```python
from build123d import *
from build123d.topology import SkipClean

# Parameters (mm, degrees)
SKETCH2_R           = 13.49375
EXTRUDE1_DEPTH      = 23.495
SKETCH15_R          = 13.4874
BOSS_EXTRUDE1_DEPTH = 17.78
SKETCH16_R          = 7.7343
CUT_EXTRUDE1_DEPTH  = 46.47293924
SKETCH20_R          = 13.4874
BOSS_EXTRUDE2_DEPTH = 17.78
SKETCH22_R          = 13.335
BOSS_EXTRUDE3_DEPTH = 21.9075
BOSS_EXTRUDE3_TAPER = 1.75
CHAMFER1_SIZE       = 1.360714286
CHAMFER1_SIZE_2     = 1.404253042
SKETCH25_R          = 13.335
BOSS_EXTRUDE4_DEPTH = 21.9075
BOSS_EXTRUDE4_DRAFT = -15
SKETCH28_R          = 10.499412296
CUT_EXTRUDE6_DEPTH  = 21.9075
FILLET1_R           = 0.762
CIRPATTERN1_COUNT   = 2
CIRPATTERN1_ANGLE   = 180
SKETCH26_R          = 7.7343
CUT_EXTRUDE4_DEPTH  = 93.597306097
SKETCH29_R          = 7.7343
CUT_EXTRUDE7_DEPTH  = 59.850524324


with BuildPart() as part:
    # Sketch2 → Extrude1 (new body)
    with BuildSketch(Plane(origin=(-41.275, 0, 0), x_dir=(0, 0, -1), z_dir=(1, 0, 0))):
        with Locations(Location((0, 0, 0), (0, 0, 180))):
            Circle(SKETCH2_R)
    extrude(amount=EXTRUDE1_DEPTH)

    # Sketch5 → Cut-Revolve1 (revolve, cut)
    with BuildSketch(Plane.XY):
        Polygon((-36.995957679, 12.118934671), (-32.762624346, 12.118934671), (-31.387809017, 13.49375), (-41.275, 13.49375), (-41.275, 8.894445), align=None)
        Polygon((-17.78, 12.118934671), (-19.896666667, 12.118934671), (-21.271481995, 13.49375), (-17.78, 13.49375), align=None)
    revolve(axis=Axis((0, 0, 0), (-1, 0, 0)), mode=Mode.SUBTRACT)

    # Sketch15 → Boss-Extrude1 (add)
    with BuildSketch(Plane(origin=(-17.78, 0, 0), x_dir=(0, 0, -1), z_dir=(1, 0, 0))):
        Circle(SKETCH15_R)
    extrude(amount=BOSS_EXTRUDE1_DEPTH)

    # Sketch16 → Cut-Extrude1 (cut, through all)
    with BuildSketch(Plane(origin=(0, 0, 0), x_dir=(0, 0, -1), z_dir=(1, 0, 0))):
        Circle(SKETCH16_R)
    extrude(amount=-CUT_EXTRUDE1_DEPTH, mode=Mode.SUBTRACT)

    # Fillet1
    fillet1_edges = [part.edges().sort_by_distance(p)[0] for p in [
        (-17.78, 0, 13.4874),
    ]]
    fillet(fillet1_edges, radius=FILLET1_R)


with BuildPart() as body_2:
    # Sketch20 → Boss-Extrude2 (new body)
    with BuildSketch(Plane(origin=(0, 17.78, 0), x_dir=(-1, 0, 0), z_dir=(0, 1, 0))):
        with Locations(Location((0, 0, 0), (0, 0, 90))):
            Circle(SKETCH20_R)
    extrude(amount=-BOSS_EXTRUDE2_DEPTH)


with BuildPart() as body_3:
    # Sketch22 → Boss-Extrude3 (new body)
    with BuildSketch(Plane(origin=(0, 17.78, 0), x_dir=(-1, 0, 0), z_dir=(0, 1, 0))):
        Circle(SKETCH22_R)
    extrude(amount=BOSS_EXTRUDE3_DEPTH, taper=BOSS_EXTRUDE3_TAPER)

    # Chamfer1
    # the kernel refuses this chamfer: 1.404253042, 1.360714286 mm, written as the material it takes off along each edge
    with BuildSketch(Plane(origin=(0, 39.6875, 0), x_dir=(-1, 0, 0), z_dir=(0, 0, 1))) as chamfer1_piece_1:
        Polygon((12.665665338 + CHAMFER1_SIZE * 0.0305385132034, CHAMFER1_SIZE * 0.999533590627), (12.665665338 - CHAMFER1_SIZE_2, 0), (12.665665338, 0), align=None)
    revolve(axis=Axis((0, 39.6875, 0), (0, -1, 0)), mode=Mode.SUBTRACT)


with BuildPart() as boss_extrude4_tool:
    # Sketch25 → Boss-Extrude4 (with draft: the straight prism first)
    with BuildSketch(Plane.XZ.offset(-17.78)):
        Circle(SKETCH25_R)
    extrude(amount=-BOSS_EXTRUDE4_DEPTH)
    # Boss-Extrude4: the draft: its side faces are tilted about the plane it starts from
    boss_extrude4_sides = [boss_extrude4_tool.faces().sort_by_distance(p)[0] for p in [
        (-13.335, 28.73375, 0),
    ]]
    draft(boss_extrude4_sides, Plane.XZ.offset(-17.78), BOSS_EXTRUDE4_DRAFT)


with BuildPart() as body_3_1:
    add(body_3.part)

    # Boss-Extrude4: add boss_extrude4_tool
    add(boss_extrude4_tool.part)

    # Sketch28 → Cut-Extrude6 (cut)
    with BuildSketch(Plane(origin=(0, 39.6875, 0), x_dir=(1, 0, 0), z_dir=(0, 1, 0))):
        with Locations(Location((0, 0, 0), (0, 0, 270))):
            Circle(SKETCH28_R)
    extrude(amount=-CUT_EXTRUDE6_DEPTH, mode=Mode.SUBTRACT)


with BuildPart() as cirpattern1_1:
    # CirPattern1: pattern copy
    add(part.part.rotate(Axis((0, 0, 12.651043997), (0, 0, -1)), 1 * CIRPATTERN1_ANGLE / (CIRPATTERN1_COUNT - 1)))


with BuildPart() as part_1:
    add(part.part)

    # Combine2: union body 3, body 2, CirPattern1_1
    add(body_3_1.part)
    add(body_2.part)
    add(cirpattern1_1.part)

    # Sketch30 → Revolve1 (revolve)
    with SkipClean():  # the faces are left unmerged after this step: merging them gives an invalid solid
        with BuildSketch(Plane.XY, mode=Mode.PRIVATE) as revolve1_sk:
            with BuildLine():
                Line((0, 17.78), (0, 8.89))
                ThreePointArc((0, 8.89), (-7.214370781, 12.4003004), (-13.589, 17.272))
                Line((-13.589, 17.272), (-13.589, 17.78))
                Line((-13.589, 17.78), (0, 17.78))
            make_face()
        revolve(revolve1_sk.sketch.rotate(Axis((0, 17.78, 0), (0, -1, 0)), 270), axis=Axis((0, 17.78, 0), (0, -1, 0)))

    # Sketch26 → Cut-Extrude4 (cut, through all)
    with SkipClean():  # the faces are left unmerged after this step: merging them gives an invalid solid
        with BuildSketch(Plane.ZY.offset(41.275)):
            with Locations(Location((0, 0, 0), (0, 0, 180))):
                Circle(SKETCH26_R)
        extrude(amount=-CUT_EXTRUDE4_DEPTH, mode=Mode.SUBTRACT)

    # Sketch29 → Cut-Extrude7 (cut, through all)
    with SkipClean():  # the faces are left unmerged after this step: merging them gives an invalid solid
        with BuildSketch(Plane(origin=(0, 0, 0), x_dir=(1, 0, 0), z_dir=(0, 1, 0))):
            with Locations(Location((0, 0, 0), (0, 0, 270))):
                Circle(SKETCH29_R)
        extrude(amount=CUT_EXTRUDE7_DEPTH, mode=Mode.SUBTRACT)


solid = part_1.part
```
Check sheet for the modelled part. Datum: model origin and axes. Units: mm. A direction names the side the tool comes from. Give positions to 0.01 mm unless a question says otherwise; leave off trailing zeros. Write each loop counter-clockwise with the first axis right and the second up, starting at its lowest first coordinate (ties: lowest second). Pieces come first, ordered by that corner, then holes.
Item 1: Cross-section at C-C (x = 24.5). Enter the section's corners in (y, z), and give its area (3 significant figures).
Item 2: Gauge pin test, flat ends, axial feed: pin 1 (3 mm diameter, centred on y = 19, z = 1.5, fed in from -X); pin 2 (8 mm diameter, centred on x = 22.5, z = -7.5, fed in from +Y); pin 3 (2 mm diameter, centred on y = 24.5, z = -9, fed in from +X). Record the tip position at first contact, or that the pin passes through.
Item 3: Cross-section at A-A (z = 0). Count the separate pieces of the cut face and the enclosed holes in it, and give its area (3 significant figures).
Item 4: Draft check along Z on faces 4 (the face through (41.275, 4, -7)), 5 (the face through (-34.85, 11.56, -3.64)), 6 (the face through (-0.58, -7.67, 1.01)), 7 (the face through (5.23, 10.74, -5.7)). Enter one of: released by +Z, released by -Z, zero draft, split by the parting line, or undercut.
Item 5: Scan lines: L1, parallel to Z at x = 0, y = 8; L2, parallel to Y at x = -10, z = 6.5; L3, parallel to Y at x = 7, z = -3.5. Record each from-to range of solid material in increasing order.
Item 6: Access from +Z, -Z, +X, -X, +Y, -Y to the whole of each face (thin tool, end or side, straight path). Record for faces 1 (the face through (26.4, 4.05, 12.87)), 2 (the face through (-26.4, -4.05, 12.87)), 3 (the face through (5.205, 17.53, 12.553)).
Item 7: Cross-section at B-B (y = 32). Enter the section's corners in (x, z).
Report:
1. outline: circle Ø26.99 at (0, 0); hole circle Ø15.47 at (0, 0)
1. area: 384 mm2
2. pin 1: stops at x = -13.57
2. pin 2: stops at y = 13.03
2. pin 3: stops at x = 10.41
3. separate pieces: 3
3. enclosed holes: 0
3. area: 925 mm2
4. face 4: zero draft
4. face 5: split by the parting line
4. face 6: undercut
4. face 7: undercut
5. L1: z = -13.49 to -7.73, 7.73 to 13.49
5. L2: y = -11.82 to -4.19, 4.19 to 39.06
5. L3: y = -13.03 to -6.9, 6.9 to 17.78
6. face 1: +X
6. face 2: -X
6. face 3: +Y
7. outline: circle Ø25.8 at (0, 0); hole circle Ø21 at (0, 0)
